from build123d import *

# Parameters (mm, degrees)
BASE_FLANGE1_DEPTH     = 0.8
SKETCHED_START         = -225
SKETCHED_BEND1_DEPTH   = 450
SKETCHED_BEND1_2_DEPTH = 450
SKETCHED_START_2       = -14.2
SKETCHED_BEND1_3_DEPTH = 16.2


with BuildPart() as part:
    # Base-Flange1: sheet metal written as solids
    # Sketch1 → Base-Flange1 (new body)
    with BuildSketch(Plane.XY):
        with BuildLine():
            Line((-29.2, 225), (29.2, 225))
            Line((29.2, 225), (29.2, -210))
            ThreePointArc((29.2, -210), (24.806601718, -220.606601718), (14.2, -225))
            Line((14.2, -225), (-14.2, -225))
            ThreePointArc((-14.2, -225), (-24.806601718, -220.606601718), (-29.2, -210))
            Line((-29.2, -210), (-29.2, 225))
        make_face()
    extrude(amount=-BASE_FLANGE1_DEPTH)

    # Sketched Bend1: read off the stored shape, not the designer's step
    # Sketched Bend1 outline → Sketched Bend1 (cut)
    with BuildSketch(Plane(origin=(0, 0, 0), x_dir=(1, 0, 0), z_dir=(0, 1, 0)).offset(SKETCHED_START)):
        with BuildLine():
            ThreePointArc((-1.099557429, 0.8), (-0.251029292, 0.587450787), (0.397105525, 0))
            Line((0.397105525, 0), (29.2, 0))
            Line((29.2, 0), (29.2, 0.8))
            Line((29.2, 0.8), (-1.099557429, 0.8))
        make_face()
    extrude(amount=SKETCHED_BEND1_DEPTH, mode=Mode.SUBTRACT)

    # Sketched Bend1 2 outline → Sketched Bend1 2 (add)
    with BuildSketch(Plane(origin=(0, 0, 0), x_dir=(1, 0, 0), z_dir=(0, 1, 0)).offset(SKETCHED_START)):
        with BuildLine():
            Line((0.700442571, -29.100442571), (0.700442571, -1))
            ThreePointArc((0.700442571, -1), (0.622939787, -0.477502784), (0.397105525, 0))
            Line((0.397105525, 0), (-1.099557429, 0))
            ThreePointArc((-1.099557429, 0), (-0.392450648, -0.292893219), (-0.099557429, -1))
            Line((-0.099557429, -1), (-0.099557429, -29.100442571))
            Line((-0.099557429, -29.100442571), (0.700442571, -29.100442571))
        make_face()
    extrude(amount=SKETCHED_BEND1_2_DEPTH)

    # Sketched Bend1 3 outline → Sketched Bend1 3 (cut)
    with BuildSketch(Plane.YZ.offset(SKETCHED_START_2)):
        with BuildLine():
            Line((-225, 29.100442571), (-225, 14.100442571))
            ThreePointArc((-225, 14.100442571), (-220.606601718, 24.707044289), (-210, 29.100442571))
            Line((-210, 29.100442571), (-225, 29.100442571))
        make_face()
    extrude(amount=SKETCHED_BEND1_3_DEPTH, mode=Mode.SUBTRACT)


solid = part.part
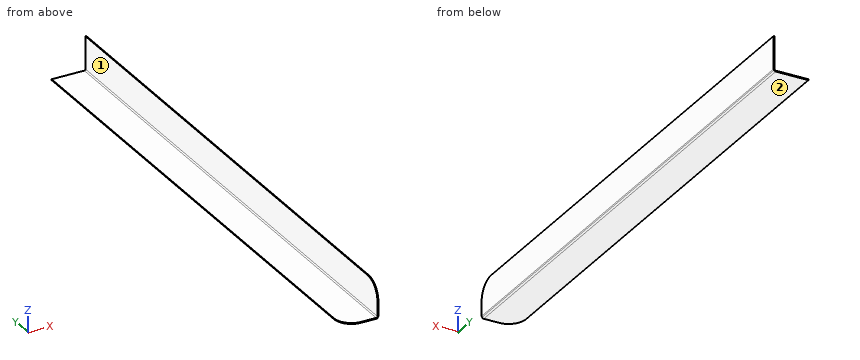
Work out the finished part from the listing and answer in its coordinate system (mm). Face numbers are marked on the shaded views. A direction names the side the tool comes from. Round coordinates to 2 decimals unless told otherwise and drop trailing zeros. Loops run counter-clockwise (first coordinate to the right, second up) from the corner with the lowest first, then second, coordinate; pieces in that order, holes last. Notation, with made-up numbers: (5.5, 45) - (18.5, 45) arc R23 cw to (18.5, 57) - close; hole circle Ø9 at (35, 40). An arc over 180 degrees is marked (long way). Use one line per item in the form item = value. Start each with the question number.
(1) A flat-ended cylindrical pin translates along its axis: P1, Ø3, axis at x = -6.5, z = 3, coming from the -Y side. Find the tip coordinate at first contact, or state that the pin passes through.
(2) Which of the six approach directions +Z, -Z, +X, -X, +Y, -Y give full straight-line access (tool end or side, diameter ignored) to the marked faces 1 and 2?
(3) Find section C-C on z = 9.75. Determine the outline of the cut face in (x, y), and give its area (3 significant figures).
(4) Find section A-A on y = -167. Determine the outline of the cut face in (x, z), and give its area (3 significant figures).
(5) Consider line 1 (Z direction, x = -2.25, y = 105); line 2 (X direction, y = -55, z = 10). Determine where each line is inside the solid, lowest interval first.
(6) Find section B-B on x = -8. Determine the outline of the cut face in (y, z).
Answer list:
q1.P1 = through
q2.face_1 = +Z, -X, +Y, -Y
q2.face_2 = -Z, +X, -X, +Y, -Y
q3.outline = (-0.1, -225) - (0.7, -225) - (0.7, 225) - (-0.1, 225) - close
q3.area = 360 mm^2
q4.outline = (-29.2, -0.8) - (-1.1, -0.8) arc R1.8 ccw to (0.7, 1) - (0.7, 29.1) - (-0.1, 29.1) - (-0.1, 1) arc R1 cw to (-1.1, 0) - (-29.2, 0) - close
q4.area = 46.7 mm^2
q5.line_1 = -0.8 to 0
q5.line_2 = -0.1 to 0.7
q6.outline = (-225, -0.8) - (225, -0.8) - (225, 0) - (-225, 0) - close
